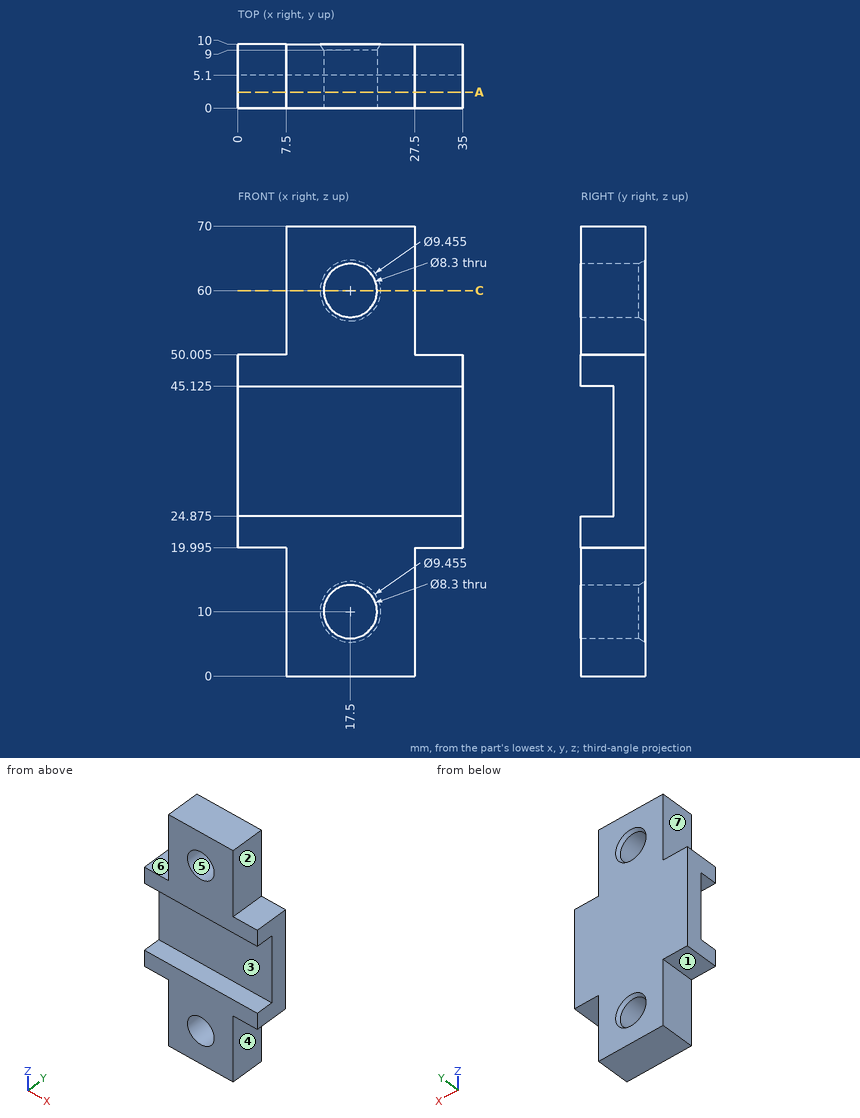
Answer from the drawing. Dimensions are ordinates in mm from the lowest x, y and z of the part. A direction names the side the tool comes from. Give positions to 0.01 mm unless a question says otherwise; leave off trailing zeros. Write each loop counter-clockwise with the first axis right and the second up, starting at its lowest first coordinate (ties: lowest second). Pieces come first, ordered by that corner, then holes.
1) Section A-A (y = 2.5) is taken. Count the separate pieces of the cut face and the enclosed holes in it, and give its area (3 significant figures).
2) A tool of negligible diameter and unlimited length cuts with its end or side. For the marked faces 1, 2 and 3, from which of +Z, -Z, +X, -X, +Y, -Y can it reach the whole face along a straight path? Write none if from no direction.
3) For a pull along X with two mould halves and no side action, classify the marked faces 4, 5, 6 and 7 as pulls with the +X half, pulls with the -X half, needs draft (parallel to the pull), parting line crosses it, or undercut.
4) Section C-C (z = 60) is taken. Write down the section's boundary in (x, y), and give its area (3 significant figures).
5) Find the intervals of material crossed by L1, parallel to Z at x = 32.5, y = 1.5 (1 decimal); L2, parallel to X at y = 3, z = 60; L3, parallel to Z at x = 26, y = 2.25 (1 decimal), in increasing order.
6) Given P1, Ø4, axis at x = 15, z = 9.5, coming from the +Y side; P2, Ø4, axis at x = 33, y = 5.5, coming from the -Z side (3 decimals); P3, Ø6, axis at x = 32.5, y = 3, coming from the +Z side (3 decimals), each flat-ended and moving along its own axis, determine where each tip first touches the part or whether it passes through.
Response:
1. separate pieces: 2
1. enclosed holes: 2
1. area: 1,030 mm2
2. face 1: -Z, -X, +Y, -Y
2. face 2: +Z, +X, +Y, -Y
2. face 3: +X, -X, -Y
3. face 4: pulls with the +X half
3. face 5: undercut
3. face 6: needs draft
3. face 7: pulls with the -X half
4. outline: (7.5, 0) - (13.35, 0) - (13.35, 9) - (12.77, 10) - (7.5, 10) - close; (21.65, 0) - (27.5, 0) - (27.5, 10) - (22.23, 10) - (21.65, 9) - close
4. area: 116 mm2
5. L1: z = 20 to 24.9, 45.1 to 50
5. L2: x = 7.5 to 13.35, 21.65 to 27.5
5. L3: z = 0 to 24.9, 45.1 to 70
6. P1: stops at y = 9.69
6. P2: stops at z = 19.995
6. P3: stops at z = 50.005
